The drawing under review shows one solid part. Ordinate dimensions are in mm from its lowest x, y, z. A direction names the side the tool comes from. Coordinates: 2 decimals unless noted, no trailing zeros. Loops run counter-clockwise (first coordinate to the right, second up) from the corner with the lowest first, then second, coordinate; pieces in that order, holes last. Notation, with made-up numbers: M 19.25,32.25 L 68.25,32.25 A24 ccw 68.25,43.25 Z; hole C -39,18 d3. An arc over 180 degrees is marked long. Use one line per item in the form item = value.
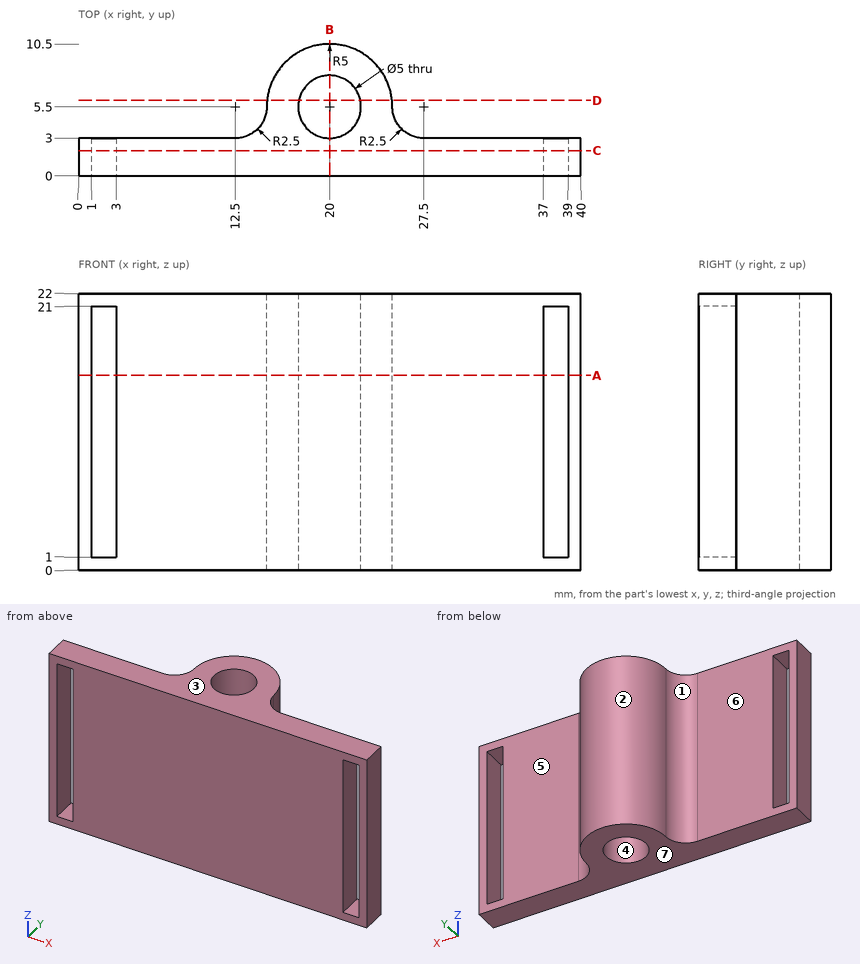
1. Consider section B-B on x = 20. Write out the cut boundary in (y, z), plus the area to 3 significant figures.
Computed values:
outline = M 0,0 L 3,0 L 3,22 L 0,22 Z; M 8,0 L 10.5,0 L 10.5,22 L 8,22 Z
area = 121 mm2
2. Wall thickness on line 1 along X through (y, z) = (2.5, 17.25); line 2 along Y through (x, z) = (20, 17.75); line 3 along Y through (x, z) = (28, 18.75): over which ranges is each line inside the solid? List them lowest first. Write a range as from..to.
Computed values:
line_1 = 0..1, 3..37, 39..40
line_2 = 0..3, 8..10.5
line_3 = 0..3
3. Consider section A-A on z = 15.5. Write out the cut boundary in (x, y).
Computed values:
outline = M 0,0 L 1,0 L 1,3 L 0,3 Z; M 3,0 L 37,0 L 37,3 L 27.5,3 A2.5 cw 25,5.5 A5 ccw 15,5.5 A2.5 cw 12.5,3 L 3,3 Z; M 39,0 L 40,0 L 40,3 L 39,3 Z; hole C 20,5.5 d5
4. Consider section D-D on y = 6. Write out the cut boundary in (x, z).
Computed values:
outline = M 15.03,0 L 17.55,0 L 17.55,22 L 15.03,22 Z; M 22.45,0 L 24.97,0 L 24.97,22 L 22.45,22 Z
5. Consider section C-C on y = 2. Write out the cut boundary in (x, z).
Computed values:
outline = M 0,0 L 40,0 L 40,22 L 0,22 Z; hole M 1,1 L 3,1 L 3,21 L 1,21 Z; hole M 37,1 L 39,1 L 39,21 L 37,21 Z
6. Draft analysis for pull direction X (two halves, no side actions). For the marked faces 1, 2, 3 and 4, state which applies: +X half, -X half, draft (parallel to the pull), parting line (faces both ways), or undercut.
Computed values:
face_1 = -X half
face_2 = parting line
face_3 = draft
face_4 = undercut
7. For pin 1 Ø6 at (x, y) = (20, 5.5) entering from -Z; pin 2 Ø10 at (x, z) = (9, 15) entering from +Y; pin 3 Ø10 at (x, z) = (35, 9.5) entering from +Y; pin 4 Ø5 at (y, z) = (6, 6.5) entering from +X, all flat-tipped, find the tip position at first contact; note any pin that passes through.
Computed values:
pin_1 = 0
pin_2 = 3.5
pin_3 = 3
pin_4 = 26
8. Tool access review of the marked faces 5, 6 and 7: name each direction out of +Z, -Z, +X, -X, +Y, -Y from which nothing blocks a thin tool from reaching the whole face with its end or side.
Computed values:
face_5 = +Z, -Z, +X, +Y
face_6 = +Z, -Z, -X, +Y
face_7 = -Z, +X, -X, +Y, -Y
